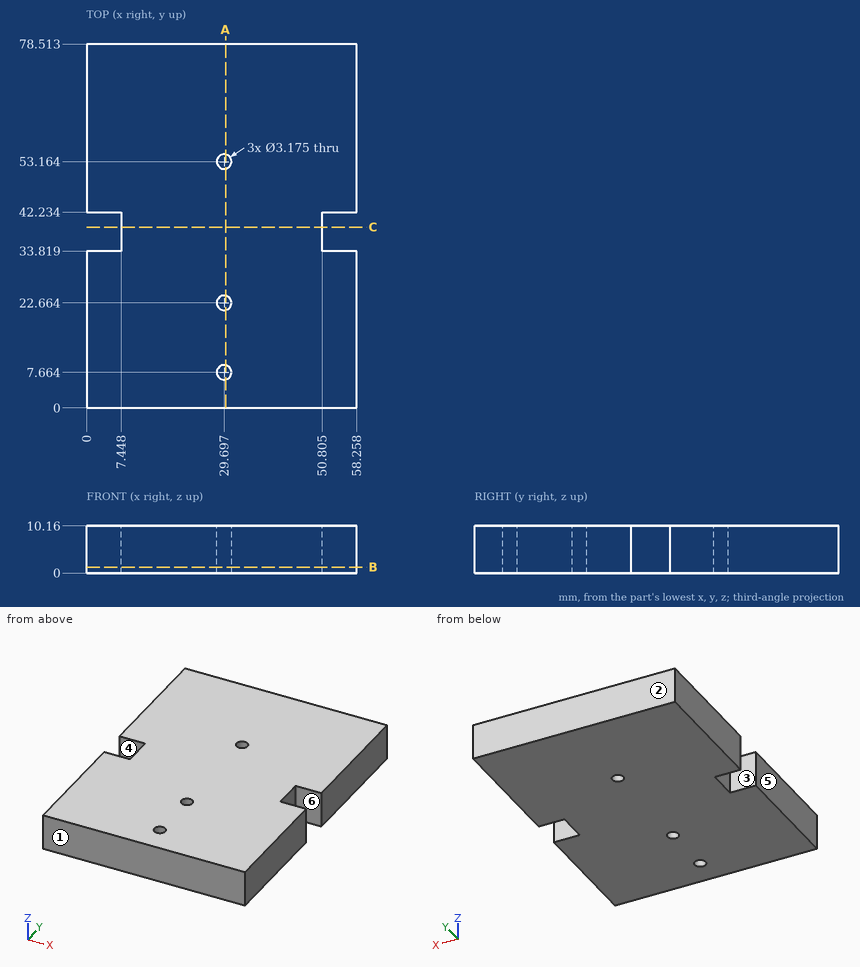
Geometry check sheet. Reference: drawing and pictorial views, mm from the part's lowest x, y, z. A direction names the side the tool comes from. Give positions to 0.01 mm unless a question says otherwise; leave off trailing zeros. Order: outer loops, then holes, each group sorted by start corner. A loop starts at its lowest first (then second) coordinate and runs counter-clockwise, first axis right, second up. Notation, with made-up numbers: (-18, 12) - (9, 12) arc R19 cw to (9, 38) - close; hole circle Ø8 at (76, -23.5). An arc over 180 degrees is marked (long way). Use one line per item in the form item = value.
1) Draft check along Y on the marked faces 1, 2 and 3. Enter one of: released by +Y, released by -Y, zero draft, split by the parting line, or undercut.
Working result:
face_1 = released by -Y
face_2 = released by +Y
face_3 = undercut
2) Material ranges on probe 1 along Y at (x, z) = (4.5, 1); probe 2 along Y at (x, z) = (29, 5) (1 decimal); probe 3 along X at (y, z) = (36.5, 1.75) (1 decimal), recorded low to high. Write a range as from..to.
Working result:
probe_1 = 0..33.82, 42.23..78.51
probe_2 = 0..6.2, 9.1..21.2, 24.1..51.7, 54.6..78.5
probe_3 = 7.4..50.8
3) Sectioned sample at A-A (x = 30). Record the boundary of the cut face in (y, z).
Working result:
outline = (0, 0) - (6.11, 0) - (6.11, 10.16) - (0, 10.16) - close; (9.22, 0) - (21.11, 0) - (21.11, 10.16) - (9.22, 10.16) - close; (24.22, 0) - (51.61, 0) - (51.61, 10.16) - (24.22, 10.16) - close; (54.72, 0) - (78.51, 0) - (78.51, 10.16) - (54.72, 10.16) - close
4) Depth check by flat-ended pin: pin 1 Ø5 at (x, y) = (29.7, 53.16) entering from +Z; pin 2 Ø4 at (y, z) = (38.5, 5) entering from +X (3 decimals). Enter the tip coordinate at first touch or a pass-through.
Working result:
pin_1 = 10.16
pin_2 = 50.805
5) Sectioned sample at C-C (y = 39). Record the boundary of the cut face in (x, z) (1 decimal).
Working result:
outline = (7.4, 0) - (50.8, 0) - (50.8, 10.2) - (7.4, 10.2) - close
6) Sectioned sample at B-B (z = 1.25). Record the boundary of the cut face in (x, y) (1 decimal), and give its area (4 significant figures).
Working result:
outline = (0, 0) - (58.3, 0) - (58.3, 33.8) - (50.8, 33.8) - (50.8, 42.2) - (58.3, 42.2) - (58.3, 78.5) - (0, 78.5) - (0, 42.2) - (7.4, 42.2) - (7.4, 33.8) - (0, 33.8) - close; hole circle Ø3.2 at (29.7, 7.7); hole circle Ø3.2 at (29.7, 22.7); hole circle Ø3.2 at (29.7, 53.2)
area = 4,425 mm^2
7) Access from +Z, -Z, +X, -X, +Y, -Y to the whole of each face (thin tool, end or side, straight path). Record for the marked faces 4, 5 and 6.
Working result:
face_4 = +Z, -Z, -X
face_5 = +Z, -Z, -X, +Y, -Y
face_6 = +Z, -Z, +X
